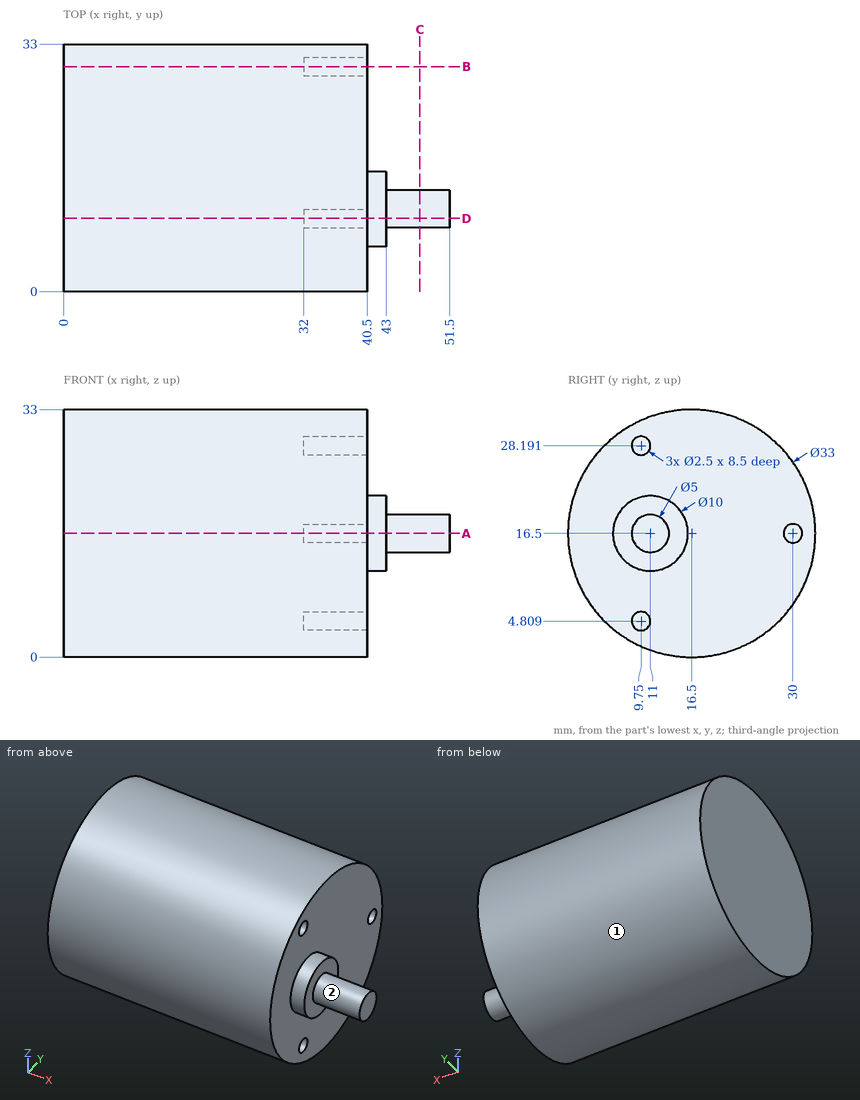
Could you check a few things on this drawing? It's one solid part, dimensions in mm from its lowest x, y, z. A direction names the side the tool comes from. Give positions to 0.01 mm unless a question says otherwise; leave off trailing zeros. Write each loop counter-clockwise with the first axis right and the second up, starting at its lowest first coordinate (ties: lowest second). Pieces come first, ordered by that corner, then holes. Notation, with made-up numbers: M 32.5,-25.5 L 38.5,-25.5 A13 ccw 38.5,-0.5 Z; hole C 58,-32 d8. An arc over 180 degrees is marked long. Put each result on its own line as item: value. Start each with the question number.
Item 1: If we section it at D-D, the plane y = 9.75: Write out the boundary of the cut face in (x, z) (1 decimal), then the cut area to 3 significant figures.
Item 2: Will these pins go through, and if not, where does the flat tip stop? pin 1 (4 mm diameter, centred on x = 25.5, y = 6.5, fed in from +Z); pin 2 (0.8 mm diameter, centred on y = 9.5, z = 4.5, fed in from +X); pin 3 (10 mm diameter, centred on x = 27, y = 7.5, fed in from +Z).
Item 3: If we section it at B-B, the plane y = 30: Write out the boundary of the cut face in (x, z).
Item 4: I need wall thicknesses on L1, parallel to Z at x = 37, y = 9; L2, parallel to X at y = 26, z = 26; L3, parallel to Y at x = 34, z = 16 (1 decimal). Which ranges of each line are inside material? Lowest first, please. Write a range as from..to.
Item 5: On a 3-axis mill with a long thin cutter (end or side, diameter ignored), from which of +Z, -Z, +X, -X, +Y, -Y can I reach the whole of each face in a straight line? I mean the marked faces 1 and 2. Say none if no direction works.
Item 6: If we section it at C-C, the plane x = 47.5: Write out the boundary of the cut face in (y, z), then the cut area to 3 significant figures.
Item 7: If we section it at A-A, the plane z = 16.5: Write out the boundary of the cut face in (x, y).
Values:
1. outline: M 0,1.4 L 40.5,1.4 L 40.5,3.6 L 32,3.6 L 32,6.1 L 40.5,6.1 L 40.5,11.7 L 43,11.7 L 43,14.3 L 51.5,14.3 L 51.5,18.7 L 43,18.7 L 43,21.3 L 40.5,21.3 L 40.5,26.9 L 32,26.9 L 32,29.4 L 40.5,29.4 L 40.5,31.6 L 0,31.6 Z
1. area: 1,240 mm²
2. pin 1: z = 30.93
2. pin 2: x = 32
2. pin 3: z = 32.51
3. outline: M 0,7.01 L 40.5,7.01 L 40.5,15.25 L 32,15.25 L 32,17.75 L 40.5,17.75 L 40.5,25.99 L 0,25.99 Z
4. L1: 1.8..3.81, 5.81..27.19, 29.19..31.2
4. L2: 0..40.5
4. L3: 0..28.9, 31.1..33
5. face 1: +X, -X
5. face 2: +X
6. outline: C 11,16.5 d5
6. area: 19.6 mm²
7. outline: M 0,0 L 40.5,0 L 40.5,6 L 43,6 L 43,8.5 L 51.5,8.5 L 51.5,13.5 L 43,13.5 L 43,16 L 40.5,16 L 40.5,28.75 L 32,28.75 L 32,31.25 L 40.5,31.25 L 40.5,33 L 0,33 Z
